Source: CAD feature listing. Evaluate the final solid. Frame: model axes, mm. Face numbers are marked on the shaded views. A direction names the side the tool comes from. Give positions to 0.01 mm unless a question says otherwise; leave off trailing zeros. Order: outer loops, then holes, each group sorted by start corner. A loop starts at its lowest first (then second) coordinate and runs counter-clockwise, first axis right, second up.
Autodesk Inventor part; units mm, degrees
ref_plane "YZ Plane" through (0, 0, 0) normal (1, 0, 0) x (0, 1, 0)
ref_plane "XZ Plane" through (0, 0, 0) normal (0, 1, 0) x (-1, 0, 0)
ref_plane "XY Plane" through (0, 0, 0) normal (0, 0, 1) x (1, 0, 0)
sketch "스케치1" plane through (0, 0, 0) normal (0, 0, 1) x (1, 0, 0)
  line L0 (0, 0) -> (0, -10)
  line L1 (0, -10) -> (77.3205, -10)
  line L2 (77.3205, -10) -> (126.9615, -38.6603)
  line L3 (126.9615, -38.6603) -> (131.9615, -30)
  line L4 (131.9615, -30) -> (80, 0)
  line L5 (80, 0) -> (0, 0)
  dimension "d0" = 10
  dimension "d1" = 80
  dimension "d2" = 60
  dimension "d4" = 150
  dimension "d5" = 10
extrude "돌출1" add sketch "스케치1" along normal mid plane 60
fillet "모깎기1" radius 8 2 edges at (0, -5, 30) (0, -5, -30)
fillet "모깎기2" radius 8 2 edges at (129.4615, -34.3301, 30) (129.4615, -34.3301, -30)
sketch "스케치2" plane through (80, 0, 30) normal (0.5, 0.866, 0) x (0.866, -0.5, 0)
  circle A0 centre (20, 30) radius 5
  circle A1 centre (40, 30) radius 5
  line L0 (60, 52) -> (60, 8)
  line L1 (52, 0) -> (0, 0)
  point P0 (-69.282, 30)
  dimension "d10" = 10
  dimension "d11" = 10
  dimension "d12" = 20
  dimension "d13" = 20
  dimension "d14" = 30
  dimension "d15" = 30
extrude "돌출2" cut sketch "스케치2" against normal blind 60
sketch "스케치3" plane through (80, 0, 30) normal (0, 1, 0) x (1, 0, 0)
  line L0 (-47.6391, 30) -> (-27.6391, 30) construction
  line L1 (-47.6391, 26) -> (-27.6391, 26)
  line L2 (-27.6391, 34) -> (-47.6391, 34)
  arc A0 (-47.6391, 34) -> (-47.6391, 26) centre (-47.6391, 30) ccw
  arc A1 (-27.6391, 26) -> (-27.6391, 34) centre (-27.6391, 30) ccw
  line L3 (-37.6391, 40) -> (-37.6391, 20) construction
  line L4 (-41.6391, 40) -> (-41.6391, 20)
  line L5 (-33.6391, 20) -> (-33.6391, 40)
  arc A2 (-33.6391, 40) -> (-41.6391, 40) centre (-37.6391, 40) ccw
  arc A3 (-41.6391, 20) -> (-33.6391, 20) centre (-37.6391, 20) ccw
  line L6 (-72, 60) -> (0, 60)
  circle A4 centre (-72, 51) radius 4
  circle A5 centre (-12, 9) radius 4
  point P0 (-80, 30)
  point P1 (-37.6391, 30)
  point P2 (-37.6391, 30)
  point P3 (-41.6391, 26)
  point P4 (-33.6391, 26)
  point P5 (-33.6391, 34)
  point P6 (-41.6391, 34)
  dimension "d18" = 20
  dimension "d19" = 20
  dimension "d20" = 30
  dimension "d21" = 30
  dimension "d22" = 8
  dimension "d23" = 8
  dimension "d24" = 60
  dimension "d25" = 42
  dimension "d26" = 9
  dimension "d28" = 8
  dimension "d29" = 8
extrude "돌출3" cut sketch "스케치3" against normal blind 60
fillet "모깎기3" radius 4 4 edges at (38.3609, -5, -4) (38.3609, -5, 4) (46.3609, -5, 4) (46.3609, -5, -4)
properties part number "2번"
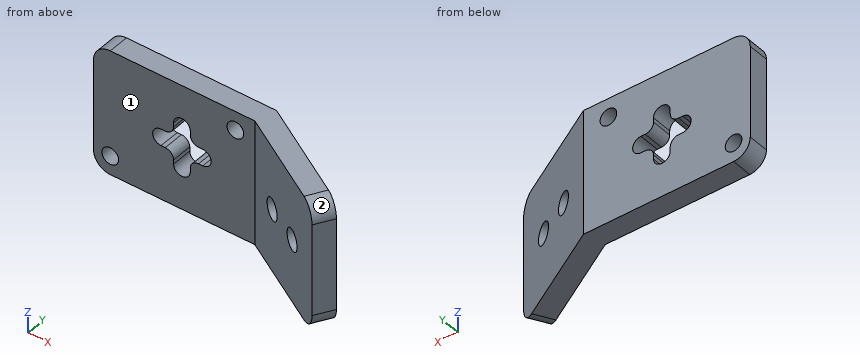
1) Section query B-B, the plane y = -4. Return the cut outline in (x, z), and give its area (3 significant figures).
Report:
outline: (0, -22) arc R8 ccw to (8, -30) - (86.93, -30) - (86.93, 30) - (8, 30) arc R8 ccw to (0, 22) - close; hole circle Ø8 at (8, -21); hole (32.36, -4) - (34.36, -4) arc R4 cw to (38.36, -8) - (38.36, -10) arc R4 ccw to (46.36, -10) - (46.36, -8) arc R4 cw to (50.36, -4) - (52.36, -4) arc R4 ccw to (52.36, 4) - (50.36, 4) arc R4 cw to (46.36, 8) - (46.36, 10) arc R4 ccw to (38.36, 10) - (38.36, 8) arc R4 cw to (34.36, 4) - (32.36, 4) arc R4 ccw to start; hole circle Ø8 at (68, 21)
area: 4,720 mm2
2) Section query C-C, the plane z = 0. Return the cut outline in (x, y), and give its area (3 significant figures).
Report:
outline: (0, -10) - (28.36, -10) - (28.36, 0) - (0, 0) - close; (56.36, -10) - (77.32, -10) - (87.99, -16.16) - (92.99, -7.5) - (80, 0) - (56.36, 0) - close; (96.65, -21.16) - (105.31, -26.16) - (110.31, -17.5) - (101.65, -12.5) - close; (113.97, -31.16) - (126.96, -38.66) - (131.96, -30) - (118.97, -22.5) - close
area: 893 mm2
3) Material intervals for L1, parallel to Z at x = 32, y = -1.5; L2, parallel to Z at x = 68, y = -3; L3, parallel to Y at x = 9.5, z = -6, sorted ascending.
Report:
L1: z = -30 to -3.98, 3.98 to 30
L2: z = -30 to 17, 25 to 30
L3: y = -10 to 0
4) Section query A-A, the plane x = 68. Return the cut outline in (y, z), and give its area (3 significant figures).
Report:
outline: (-10, -30) - (0, -30) - (0, 17) - (-10, 17) - close; (-10, 25) - (0, 25) - (0, 30) - (-10, 30) - close
area: 520 mm2
5) Reachability of the marked faces 1 and 2 from +Z, -Z, +X, -X, +Y, -Y: full face, straight path, thin tool, end or side. Return the list, or none.
Report:
face 1: +Z, -Z, -X, -Y
face 2: +Z, +X, -Y
6) Pin query (flat end, axial travel): pin 1 (4 mm diameter, centred on x = 95.5, y = -6, fed in from +Z); pin 2 (2 mm diameter, centred on x = 84, z = 0, fed in from -Y); pin 3 (10 mm diameter, centred on x = 93.5, z = 7, fed in from -Y); pin 4 (13 mm diameter, centred on x = 68, z = 21, fed in from -Y). Return the tip coordinate at first contact, or that it passes through.
Report:
pin 1: passes through
pin 2: stops at y = -14.43
pin 3: stops at y = -22.23
pin 4: stops at y = -10
7) Section query D-D, the plane x = 22.5. Return the cut outline in (y, z).
Report:
outline: (-10, -30) - (0, -30) - (0, 30) - (-10, 30) - close
